Check sheet for the modelled part. Datum: model origin and axes. Units: mm. Coordinates: 2 decimals unless noted, no trailing zeros. Loops run counter-clockwise (first coordinate to the right, second up) from the corner with the lowest first, then second, coordinate; pieces in that order, holes last. Notation, with made-up numbers: (79, 26.25) -> (98, 26.25) arc R12 ccw to (98, 41.25) -> close; hole circle Ø10 at (81.25, 67.5). An arc over 180 degrees is marked (long way). Use CSV: the item, a comma, the result in double quotes.
```python
from build123d import *

# Parameters (mm, degrees)
SKETCH4_R           = 2.5
SKETCH4_R_2         = 1.8415
BOSS_EXTRUDE4_DEPTH = 7.5
SKETCH5_W           = 97.316999936
SKETCH5_H           = 58.277
SKETCH5_W_2         = 88.78146603
SKETCH5_H_2         = 49.741466094
BOSS_EXTRUDE5_DEPTH = 2


with BuildPart() as part:
    # Sketch4 → Boss-Extrude4 (new body)
    with BuildSketch(Plane(origin=(0, 0, 0), x_dir=(1, 0, 0), z_dir=(0, 1, 0))):
        with Locations(Location((92.6585, 62.6915, 0), (0, 0, 270))):
            Circle(SKETCH4_R)
        with Locations((92.6585, 62.6915)):
            Circle(SKETCH4_R_2, mode=Mode.SUBTRACT)
        with Locations((92.6585, 62.6915)):
            Circle(SKETCH4_R_2)
        with Locations(Location((0.341500064, 62.6915, 0), (0, 0, 270))):
            Circle(SKETCH4_R)
        with Locations((0.341500064, 62.6915)):
            Circle(SKETCH4_R_2, mode=Mode.SUBTRACT)
        with Locations((0.341500064, 62.6915)):
            Circle(SKETCH4_R_2)
        with Locations(Location((0.341500064, 115.9685, 0), (0, 0, 270))):
            Circle(SKETCH4_R)
        with Locations((0.341500064, 115.9685)):
            Circle(SKETCH4_R_2, mode=Mode.SUBTRACT)
        with Locations((0.341500064, 115.9685)):
            Circle(SKETCH4_R_2)
        with Locations(Location((92.6585, 115.9685, 0), (0, 0, 270))):
            Circle(SKETCH4_R)
        with Locations((92.6585, 115.9685)):
            Circle(SKETCH4_R_2, mode=Mode.SUBTRACT)
        with Locations((92.6585, 115.9685)):
            Circle(SKETCH4_R_2)
    extrude(amount=BOSS_EXTRUDE4_DEPTH)

    # Sketch5 → Boss-Extrude5 (add)
    with BuildSketch(Plane.XZ):
        with Locations((46.500000032, -89.33)):
            Rectangle(SKETCH5_W, SKETCH5_H)
        with Locations((46.500000032, -89.33)):
            Rectangle(SKETCH5_W_2, SKETCH5_H_2, mode=Mode.SUBTRACT)
    extrude(amount=-BOSS_EXTRUDE5_DEPTH)


solid = part.part
```
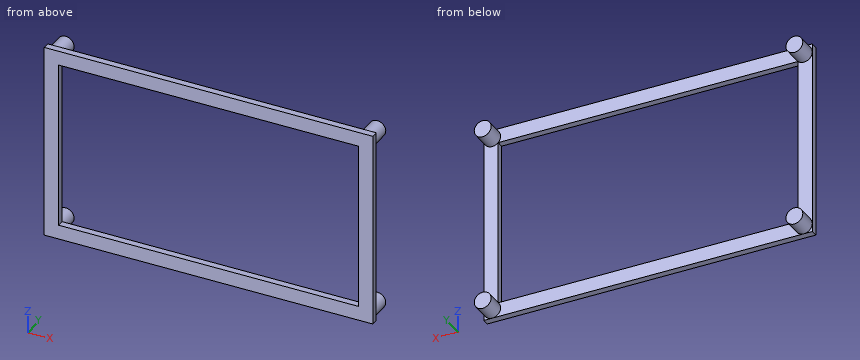
1) Cross-section at B-B on z = -101. Record the boundary of the cut face in (x, y), and give its area (3 significant figures).
Answer below:
outline,"(-2.16, 0) -> (2.11, 0) -> (2.11, 2) -> (-2.16, 2) -> close; (90.89, 0) -> (95.16, 0) -> (95.16, 2) -> (90.89, 2) -> close"
area,"17.1 mm²"
2) Cross-section at A-A on x = 8. Record the boundary of the cut face in (y, z), and give its area (3 significant figures).
Answer below:
outline,"(0, -118.47) -> (2, -118.47) -> (2, -114.2) -> (0, -114.2) -> close; (0, -64.46) -> (2, -64.46) -> (2, -60.19) -> (0, -60.19) -> close"
area,"17.1 mm²"
3) Go/stop test with a flat-tipped pin: pin 1 Ø2 at (x, z) = (-0.5, -77.5) entering from +Y. Record where the tip stops, or that it passes through.
Answer below:
pin 1,"stops at y = 2"
4) Thickness scan on line 1 along Z through (x, y) = (75.5, 0.5); line 2 along X through (y, z) = (1.25, -66.5). Record the ranges inside material, lowest first. Write a range as from..to.
Answer below:
line 1,"z = -118.47..-114.2, -64.46..-60.19"
line 2,"x = -2.16..2.11, 90.89..95.16"
5) Cross-section at C-C on y = 5. Record the boundary of the cut face in (x, z).
Answer below:
outline,"circle Ø5 at (0.34, -115.97); circle Ø5 at (0.34, -62.69); circle Ø5 at (92.66, -115.97); circle Ø5 at (92.66, -62.69)"
